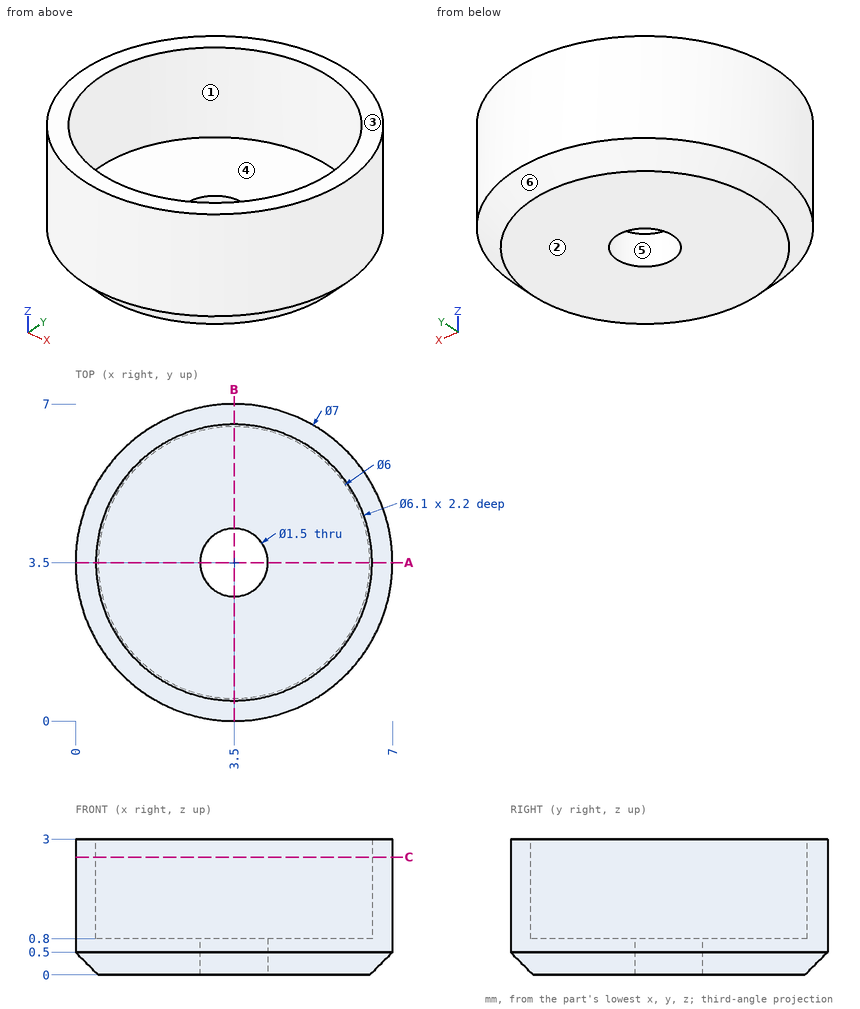
Check sheet for the drawn part. Datum: minimum x, y, z corner. Units: mm. A direction names the side the tool comes from. Round coordinates to 2 decimals unless told otherwise and drop trailing zeros. Write each loop counter-clockwise with the first axis right and the second up, starting at its lowest first coordinate (ties: lowest second). Pieces come first, ordered by that corner, then holes. Notation, with made-up numbers: (27, 55) - (58, 55) arc R36 cw to (58, 89) - close; hole circle Ø10 at (-22, 13.5). An arc over 180 degrees is marked (long way). Write each question's results on one line, items separated by ' | '.
(1) Sectioned sample at A-A, the plane y = 3.5. Enter the section's corners in (x, z), plus the area to 3 significant figures.
Computed:
outline: (0, 0.5) - (0.5, 0) - (2.75, 0) - (2.75, 0.8) - (0.45, 0.8) - (0.45, 3) - (0, 3) - close; (4.25, 0) - (6.5, 0) - (7, 0.5) - (7, 3) - (6.55, 3) - (6.55, 0.8) - (4.25, 0.8) - close | area: 6.13 mm^2
(2) Sectioned sample at C-C, the plane z = 2.6. Enter the section's corners in (x, y), plus the area to 3 significant figures.
Computed:
outline: circle Ø7 at (3.5, 3.5); hole circle Ø6.1 at (3.5, 3.5) | area: 9.26 mm^2
(3) Thickness scan on probe 1 along Y at (x, z) = (3.5, 2.1); probe 2 along Y at (x, z) = (3.5, 0.6); probe 3 along X at (y, z) = (1.75, 2.65). Record the ranges inside material, lowest first. Write a range as from..to.
Computed:
probe 1: y = 0..0.45, 6.55..7 | probe 2: y = 0..2.75, 4.25..7 | probe 3: x = 0.47..1, 6..6.53
(4) Draft check along Y on the marked faces 3, 4, 5 and 6. Enter one of: pulls with the +Y half, pulls with the -Y half, needs draft (parallel to the pull), parting line crosses it, or undercut.
Computed:
face 3: needs draft | face 4: undercut | face 5: undercut | face 6: parting line crosses it
(5) Depth check by flat-ended pin: pin 1 Ø1.4 at (x, y) = (3.5, 3.5) entering from -Z; pin 2 Ø1 at (y, z) = (3, 1) entering from +X; pin 3 Ø1 at (x, y) = (4, 4) entering from +Z. Enter the tip coordinate at first touch or a pass-through.
Computed:
pin 1: passes through | pin 2: stops at x = 7 | pin 3: stops at z = 0.8
(6) Set-up check for the marked faces 1 and 2: record each of +Z, -Z, +X, -X, +Y, -Y from which the full face is reachable in a straight line by a thin tool's end or side.
Computed:
face 1: +Z | face 2: -Z, +X, -X, +Y, -Y
